```python
from build123d import *

# Parameters (mm, degrees)
SKETCH_3_W               = 20
SKETCH_3_H               = 20
EXTRUDE_1_DEPTH          = 500
SKETCH_6_W               = 16
SKETCH_6_H               = 16
CUT_EXTRUDE_3_DEPTH      = 560
SKETCH_8_W               = 20
SKETCH_8_H               = 20
SKETCH_8_W_2             = 16
SKETCH_8_H_2             = 16
EXTRUDE_3_DEPTH          = 20
SKETCH_12_R              = 1
CUT_EXTRUDE_7_DEPTH      = 10
M4X0_7_1_D               = 3.3
M4X0_7_1_DEPTH           = 11.5
M4X0_7_1_TIP             = 0.991420021
M4X0_7_1_ON_FACE_2_D     = 3.3
M4X0_7_1_ON_FACE_2_DEPTH = 11.5
M4X0_7_1_ON_FACE_2_TIP   = 0.991420021


with BuildPart() as part:
    # ｽｹｯﾁ3 → ﾎﾞｽ - 押し出し1 (new body)
    with BuildSketch(Plane.XY):
        Rectangle(SKETCH_3_W, SKETCH_3_H)
    extrude(amount=EXTRUDE_1_DEPTH)

    # ｽｹｯﾁ6 → ｶｯﾄ - 押し出し3 (cut)
    with BuildSketch(Plane.XY.offset(500)):
        Rectangle(SKETCH_6_W, SKETCH_6_H)
    extrude(amount=-CUT_EXTRUDE_3_DEPTH, mode=Mode.SUBTRACT)

    # ｽｹｯﾁ8 → ﾎﾞｽ - 押し出し3 (add)
    with BuildSketch(Plane.XY.offset(500)):
        Rectangle(SKETCH_8_W, SKETCH_8_H)
        Rectangle(SKETCH_8_W_2, SKETCH_8_H_2, mode=Mode.SUBTRACT)
    extrude(amount=EXTRUDE_3_DEPTH)

    # ｽｹｯﾁ12 → ｶｯﾄ - 押し出し7 (cut)
    with BuildSketch(Plane.ZY.offset(10)):
        with Locations((20, 0)):
            Circle(SKETCH_12_R)
        with Locations((500, 0)):
            Circle(SKETCH_12_R)
    extrude(amount=-CUT_EXTRUDE_7_DEPTH, mode=Mode.SUBTRACT)

    # M4x0.7 ねじ穴1
    with Locations(Plane(origin=(-10, 0, 20), x_dir=(0, -1, 0), z_dir=(-1, 0, 0))):
        with Locations((0, 0)):
            Hole(M4X0_7_1_D / 2, depth=M4X0_7_1_DEPTH)
            with Locations((0, 0, -(M4X0_7_1_DEPTH + M4X0_7_1_TIP / 2))):  # 118° drill point
                Cone(0, M4X0_7_1_D / 2, M4X0_7_1_TIP, mode=Mode.SUBTRACT)

    # M4x0.7 ねじ穴1 on face 2
    with Locations(Plane(origin=(-8, 0, 500), x_dir=(0, -1, 0), z_dir=(-1, 0, 0))):
        with Locations((0, 0)):
            Hole(M4X0_7_1_ON_FACE_2_D / 2, depth=M4X0_7_1_ON_FACE_2_DEPTH)
            with Locations((0, 0, -(M4X0_7_1_ON_FACE_2_DEPTH + M4X0_7_1_ON_FACE_2_TIP / 2))):  # 118° drill point
                Cone(0, M4X0_7_1_ON_FACE_2_D / 2, M4X0_7_1_ON_FACE_2_TIP, mode=Mode.SUBTRACT)


solid = part.part
```
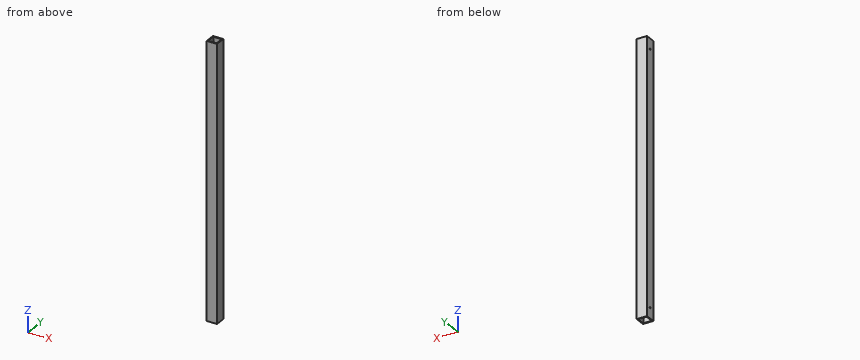
Source: CAD feature listing. Evaluate the final solid. Frame: model axes, mm. Coordinates: 2 decimals unless noted, no trailing zeros. Write each loop counter-clockwise with the first axis right and the second up, starting at its lowest first coordinate (ties: lowest second). Pieces come first, ordered by that corner, then holes. Notation, with made-up numbers: (39.25, -2.75) -> (63.25, -2.75) arc R21 cw to (63.25, 30.25) -> close; hole circle Ø2 at (57, 67). An arc over 180 degrees is marked (long way). Return JSON: item names as keys, results as strings. Group by question number.
1) Ray query, line 1 along Z through (x, y) = (-9.2, 0); line 2 along Y through (x, z) = (5.75, 428); line 3 along Y through (x, z) = (-8.5, 500). Return the intervals inside material, ascending.
2) Section query A-A, the plane x = -0.5. Return loops of the section in (y, z), plus the area to 3 significant figures.
3) Contact query for a flat-ended pin moving along its axis: P1, Ø3, axis at y = 0, z = 20, coming from the -X side. Output: stop coordinate, or through.
4) Section query B-B, the plane z = 104. Return loops of the section in (x, y).
From the geometry:
{
 "1": {"line 1": "0 to 18.35, 21.65 to 498.35, 501.65 to 520", "line 2": "-10 to -8, 8 to 10", "line 3": "-10 to -1.65, 1.65 to 10"},
 "2": {"outline": "(-10, 0) -> (-8, 0) -> (-8, 520) -> (-10, 520) -> close; (8, 0) -> (10, 0) -> (10, 520) -> (8, 520) -> close", "area": "2,080 mm²"},
 "3": {"P1": "x = 8"},
 "4": {"outline": "(-10, -10) -> (10, -10) -> (10, 10) -> (-10, 10) -> close; hole (-8, -8) -> (8, -8) -> (8, 8) -> (-8, 8) -> close"}
}
